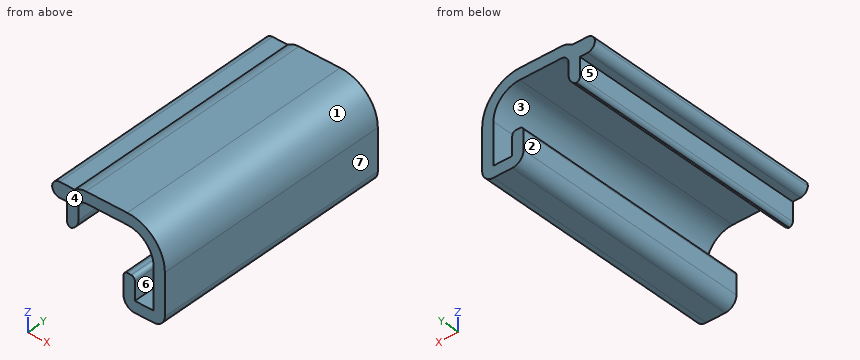
```python
from build123d import *

# Parameters (mm, degrees)
F1_DEPTH    = 65
F2_R        = 1
F3_R        = 1.99999
F4_T1_DEPTH = 79.1421356237


# Not quite as in the source:
# - a fillet or chamfer that OpenCascade refuses, or shapes differently, is made with other operations: its cross-section is extruded or revolved along the edge and cut away or added
# - a fillet or chamfer is up to 0.001 mm smaller than in the source, because OpenCascade refuses the exact size
# - a feature names something its author has since deleted; it is built from what else it names


with BuildPart() as f1:
    # F0 (on Front) → F1 (new body)
    with BuildSketch(Plane.XZ):
        with BuildLine():
            ThreePointArc((0, -2), (0.5857864376, -0.5857864376), (2, 0))
            Line((2, 0), (13, 0))
            ThreePointArc((13, 0), (17.9497474683, -2.0502525317), (20, -7))
            Line((20, -7), (20, -18))
            Line((20, -18), (15, -18))
            Line((15, -18), (15, -12))
            Line((15, -12), (12, -12))
            Line((12, -12), (12, -18))
            ThreePointArc((12, -18), (12.8786796564, -20.1213203436), (15, -21))
            Line((15, -21), (20, -21))
            ThreePointArc((20, -21), (22.1213203436, -20.1213203436), (23, -18))
            Line((23, -18), (23, -7))
            ThreePointArc((23, -7), (20.0710678119, 0.0710678119), (13, 3))
            Line((13, 3), (2, 3))
            ThreePointArc((2, 3), (0.4188611699, 2.7434164903), (-1, 2))
            ThreePointArc((-1, 2), (-2.472135955, 0.2360679775), (-3, -2))
            Line((-3, -2), (-3, -8))
            Line((-3, -8), (0, -8))
            Line((0, -8), (0, -2))
        make_face()
        with BuildLine():
            Line((-7, -2), (-3, -2))
            ThreePointArc((-3, -2), (-2.472135955, 0.2360679775), (-1, 2))
            Line((-1, 2), (-7, 2))
            Line((-7, 2), (-7, -2))
        make_face()
    extrude(amount=F1_DEPTH)

    # F2
    f2_edges = [f1.edges().sort_by_distance(p)[0] for p in [
        (-3, -32.5, -8),
        (12, -32.5, -12),
        (15, -32.5, -12),
    ]]
    fillet(f2_edges, radius=F2_R)

    # F3 (radius 2 in the source; OpenCascade refuses exactly that, so slightly less here)
    f3_edges = [f1.edges().sort_by_distance(p)[0] for p in [
        (-7, -32.5, -2),
        (-7, -32.5, 2),
    ]]
    fillet(f3_edges, radius=F3_R)

    # F4: fillet of radius 3 on 1 edges, made by hand

    # F4_s2 → F4_t1 (cut)
    with BuildSketch(Plane.XZ.offset(-7.0710678119)):
        with BuildLine():
            ThreePointArc((-2, -8), (-0.5505102572, -6.9036236828), (0, -5.1715728753))
            Line((0, -5.1715728753), (0.06, -5.1715728753))
            Line((0.06, -5.1715728753), (0.06, -8))
            Line((0.06, -8), (0, -8.06))
            ThreePointArc((0, -8.06), (-1, -8.06), (-1.98, -8.0565685425))
            Line((-1.98, -8.0565685425), (-2, -8))
        make_face()
    extrude(amount=F4_T1_DEPTH, mode=Mode.SUBTRACT)


solid = f1.part
```
Verification items for the finished model (mm, model axes). Face numbers are marked on the shaded views. A direction names the side the tool comes from. Round coordinates to 2 decimals unless told otherwise and drop trailing zeros. Write each loop counter-clockwise with the first axis right and the second up, starting at its lowest first coordinate (ties: lowest second). Pieces come first, ordered by that corner, then holes. Notation, with made-up numbers: (35.5, 55) -> (81.5, 55) arc R27 ccw to (81.5, 86) -> close; hole circle Ø10 at (85.5, 50). An arc over 180 degrees is marked (long way). Write each question's results on one line, items separated by ' | '. Start each with the question number.
1. Cross-section at C-C (x = 18.5). Enter the section's corners in (y, z), then the cut area to 3 significant figures.
2. Material ranges on probe 1 along X at (y, z) = (-35.5, -14.5); probe 2 along X at (y, z) = (-33, -3.75); probe 3 along X at (y, z) = (-34, -9.5), recorded low to high. Write a range as from..to.
3. Cross-section at A-A (z = -15.25). Enter the section's corners in (x, y).
4. Depth check by flat-ended pin: P1, Ø1.5, axis at y = -29.5, z = -16.5, coming from the -X side; P2, Ø2.5, axis at x = 18, y = -19.5, coming from the +Z side; P3, Ø1.5, axis at x = 17, y = -11.5, coming from the +Z side. Enter the tip coordinate at first touch or a pass-through.
5. Cross-section at D-D (x = 6.75). Enter the section's corners in (y, z), then the cut area to 3 significant figures.
6. Draft check along X on the marked faces 1, 2, 3 and 4. Enter one of: +X half, -X half, draft (parallel to the pull), parting line (faces both ways), or undercut.
7. Set-up check for the marked faces 5, 6 and 7: record each of +Z, -Z, +X, -X, +Y, -Y from which the full face is reachable in a straight line by a thin tool's end or side.
Solutions:
1) outline: (-65, -21) -> (0, -21) -> (0, -18) -> (-65, -18) -> close; (-65, -2.67) -> (0, -2.67) -> (0, 1.35) -> (-65, 1.35) -> close | area: 456 mm2
2) probe 1: x = 12..15, 20..23 | probe 2: x = -3..0, 19.2..22.46 | probe 3: x = 20..23
3) outline: (12, -65) -> (15, -65) -> (15, 0) -> (12, 0) -> close; (20, -65) -> (23, -65) -> (23, 0) -> (20, 0) -> close
4) P1: stops at x = 12 | P2: stops at z = 2.27 | P3: stops at z = 2.46
5) outline: (-65, 0) -> (0, 0) -> (0, 3) -> (-65, 3) -> close | area: 195 mm2
6) face 1: +X half | face 2: -X half | face 3: undercut | face 4: draft
7) face 5: -Z, -X, +Y, -Y | face 6: +Y, -Y | face 7: +Z, -Z, +X, +Y, -Y
